from build123d import *

# Parameters (mm, degrees)
SKETCH1_R           = 3.3782
BOSS_EXTRUDE1_DEPTH = 3.175
SKETCH4_W           = 23.114
SKETCH4_H           = 213.36
CUT_EXTRUDE1_DEPTH  = 263.804276362
FILLET1_R           = 17.78
FILLET2_R           = 35.56


with BuildPart() as part:
    # Sketch1 → Boss-Extrude1 (new body)
    with BuildSketch(Plane(origin=(0, 0, 0), x_dir=(1, 0, 0), z_dir=(0, 1, 0))):
        Polygon((-240.157, 106.68), (240.157, 106.68), (240.157, -73.66), (240.157, -106.68), (-240.157, -106.68), align=None)
        with Locations(Location((224.282, -73.66, 0), (0, 0, 270))):
            Circle(SKETCH1_R, mode=Mode.SUBTRACT)
        with Locations(Location((-21.7805, -90.805, 0), (0, 0, 270))):
            Circle(SKETCH1_R, mode=Mode.SUBTRACT)
        with Locations(Location((-21.7805, 90.805, 0), (0, 0, 90))):
            Circle(SKETCH1_R, mode=Mode.SUBTRACT)
        with Locations(Location((224.282, 73.66, 0), (0, 0, 90))):
            Circle(SKETCH1_R, mode=Mode.SUBTRACT)
        with Locations(Location((-115.697, 93.98, 0), (0, 0, 270))):
            Circle(SKETCH1_R, mode=Mode.SUBTRACT)
        with Locations(Location((-115.697, -93.98, 0), (0, 0, 90))):
            Circle(SKETCH1_R, mode=Mode.SUBTRACT)
        with Locations(Location((-181.737, 71.12, 0), (0, 0, 270))):
            Circle(SKETCH1_R, mode=Mode.SUBTRACT)
        with Locations(Location((-49.657, 71.12, 0), (0, 0, 270))):
            Circle(SKETCH1_R, mode=Mode.SUBTRACT)
        with Locations(Location((-49.657, -71.12, 0), (0, 0, 90))):
            Circle(SKETCH1_R, mode=Mode.SUBTRACT)
        with Locations(Location((-181.737, -71.12, 0), (0, 0, 90))):
            Circle(SKETCH1_R, mode=Mode.SUBTRACT)
        with BuildLine():
            Line((119.507, -19.4818), (208.407, -19.4818))
            ThreePointArc((208.407, -19.4818), (211.7852, -22.86), (208.407, -26.2382))
            Line((208.407, -26.2382), (119.507, -26.2382))
            ThreePointArc((119.507, -26.2382), (116.1288, -22.86), (119.507, -19.4818))
        make_face(mode=Mode.SUBTRACT)
        with BuildLine():
            Line((119.507, 19.4818), (208.407, 19.4818))
            ThreePointArc((208.407, 19.4818), (211.7852, 22.86), (208.407, 26.2382))
            Line((208.407, 26.2382), (119.507, 26.2382))
            ThreePointArc((119.507, 26.2382), (116.1288, 22.86), (119.507, 19.4818))
        make_face(mode=Mode.SUBTRACT)
        with BuildLine():
            Line((127.762, -57.5818), (206.502, -57.5818))
            ThreePointArc((206.502, -57.5818), (209.8802, -60.96), (206.502, -64.3382))
            Line((206.502, -64.3382), (127.762, -64.3382))
            ThreePointArc((127.762, -64.3382), (124.3838, -60.96), (127.762, -57.5818))
        make_face(mode=Mode.SUBTRACT)
        with BuildLine():
            Line((127.762, -89.7382), (206.502, -89.7382))
            ThreePointArc((206.502, -89.7382), (209.8802, -86.36), (206.502, -82.9818))
            Line((206.502, -82.9818), (127.762, -82.9818))
            ThreePointArc((127.762, -82.9818), (124.3838, -86.36), (127.762, -89.7382))
        make_face(mode=Mode.SUBTRACT)
        with BuildLine():
            Line((127.762, 57.5818), (206.502, 57.5818))
            ThreePointArc((206.502, 57.5818), (209.8802, 60.96), (206.502, 64.3382))
            Line((206.502, 64.3382), (127.762, 64.3382))
            ThreePointArc((127.762, 64.3382), (124.3838, 60.96), (127.762, 57.5818))
        make_face(mode=Mode.SUBTRACT)
        with BuildLine():
            Line((127.762, 89.7382), (206.502, 89.7382))
            ThreePointArc((206.502, 89.7382), (209.8802, 86.36), (206.502, 82.9818))
            Line((206.502, 82.9818), (127.762, 82.9818))
            ThreePointArc((127.762, 82.9818), (124.3838, 86.36), (127.762, 89.7382))
        make_face(mode=Mode.SUBTRACT)
        with BuildLine():
            Line((5.207, 3.3782), (30.607, 3.3782))
            ThreePointArc((30.607, 3.3782), (33.9852, 0), (30.607, -3.3782))
            Line((30.607, -3.3782), (5.207, -3.3782))
            ThreePointArc((5.207, -3.3782), (1.8288, 0), (5.207, 3.3782))
        make_face(mode=Mode.SUBTRACT)
    extrude(amount=BOSS_EXTRUDE1_DEPTH)

    # Sketch4 → Cut-Extrude1 (cut, through all)
    with BuildSketch(Plane(origin=(0, 3.175, 0), x_dir=(1, 0, 0), z_dir=(0, 1, 0))):
        with Locations((-228.6, 0)):
            Rectangle(SKETCH4_W, SKETCH4_H)
    extrude(amount=-CUT_EXTRUDE1_DEPTH, mode=Mode.SUBTRACT)

    # Fillet1
    fillet1_edges = [part.edges().sort_by_distance(p)[0] for p in [
        (240.157, 1.5875, 106.68),
        (240.157, 1.5875, -106.68),
    ]]
    fillet(fillet1_edges, radius=FILLET1_R)

    # Fillet2
    fillet2_edges = [part.edges().sort_by_distance(p)[0] for p in [
        (-217.043, 1.5875, -106.68),
        (-217.043, 1.5875, 106.68),
    ]]
    fillet(fillet2_edges, radius=FILLET2_R)


solid = part.part
Geometry: final body of the model. Coordinates: model frame, mm. Give positions to 0.01 mm unless a question says otherwise; leave off trailing zeros. Loops run counter-clockwise (first coordinate to the right, second up) from the corner with the lowest first, then second, coordinate; pieces in that order, holes last. Notation, with made-up numbers: (85.25, -24.75) - (96.25, -24.75) arc R11 cw to (96.25, -14.75) - close; hole circle Ø3 at (45, 66.5). An arc over 180 degrees is marked (long way). One line per question, with ' | ' between items. Start each with the question number.
(1) Section query A-A on x = 20. Return loops of the section in (y, z) (3 decimals).
(2) Section query C-C on y = 0.85. Count the separate pieces of the cut face and the enclosed holes in it, then the cut area to 3 significant figures.
(3) Section query B-B on x = 194.5. Return loops of the section in (y, z) (3 decimals), then the cut area to 3 significant figures.
(4) Contact query for flat-ended pins moving along their axis: pin 1 (1.5 mm diameter, centred on x = 11.5, z = 34.5, fed in from -Y); pin 2 (1 mm diameter, centred on y = 1.5, z = -73.5, fed in from -X). Output: stop coordinate, or through.
(5) Ray query, line 1 (X direction, y = 1.7, z = 73.66); line 2 (Z direction, x = 11.5, y = 0.95); line 3 (X direction, y = 2.2, z = -71.12). Return the intervals inside material, ascending. Write a range as from..to.
The answers:
1) outline: (0, -106.68) - (3.175, -106.68) - (3.175, -3.378) - (0, -3.378) - close; (0, 3.378) - (3.175, 3.378) - (3.175, 106.68) - (0, 106.68) - close
2) separate pieces: 1 | enclosed holes: 17 | area: 92,800 mm2
3) outline: (0, -106.68) - (3.175, -106.68) - (3.175, -89.738) - (0, -89.738) - close; (0, -82.982) - (3.175, -82.982) - (3.175, -64.338) - (0, -64.338) - close; (0, -57.582) - (3.175, -57.582) - (3.175, -26.238) - (0, -26.238) - close; (0, -19.482) - (3.175, -19.482) - (3.175, 19.482) - (0, 19.482) - close; (0, 26.238) - (3.175, 26.238) - (3.175, 57.582) - (0, 57.582) - close; (0, 64.338) - (3.175, 64.338) - (3.175, 82.982) - (0, 82.982) - close; (0, 89.738) - (3.175, 89.738) - (3.175, 106.68) - (0, 106.68) - close | area: 549 mm2
4) pin 1: y = 0 | pin 2: x = -216.99
5) line 1: -216.95..-183.96, -179.51..-51.88, -47.43..220.9, 227.66..240.16 | line 2: -106.68..-3.38, 3.38..106.68 | line 3: -217.04..-185.12, -178.36..-53.04, -46.28..222.05, 226.51..240.16
